from build123d import *

# Parameters (mm, degrees)
F0_R       = 17.0692141661
F1_DEPTH   = 74.676
F3_DEPTH   = 7.62
F1_FACE1_R = 17.0692141661
F5_DEPTH   = 8.128
F7_DEPTH   = 14.732
F9_DEPTH   = 14.478
F10_R      = 6.1442753349
F11_DEPTH  = 157.481
F12_R      = 6.3140721671
F13_DEPTH  = 157.481


with BuildPart() as f1:
    # F0 (on Right) → F1 (new body, symmetric)
    with BuildSketch(Plane.YZ):
        with Locations((0, -44.9254028499)):
            Circle(F0_R)
    extrude(amount=F1_DEPTH, both=True)

    # F2 (on face) → F3 (join)
    with BuildSketch(Plane.YZ.offset(74.676)):
        with BuildLine():
            ThreePointArc((17.0692141661, -44.9254028499), (17.054567773, -45.6323613518), (17.0106537288, -46.3381066294))
            Line((17.0106537288, -46.3381066294), (17.6849197596, -46.3381066294))
            Line((17.6849197596, -46.3381066294), (17.6849197596, 24.6733147651))
            Line((17.6849197596, 24.6733147651), (-17.0106537288, 24.6733147651))
            Line((-17.0106537288, 24.6733147651), (-17.0106537288, -43.5126990704))
            ThreePointArc((-17.0106537288, -43.5126990704), (0.7069585019, -27.8708350769), (17.0692141661, -44.9254028499))
        make_face()
    extrude(amount=-F3_DEPTH)

    # F4 (on face) + F1_face1 (on face) → F5 (join)
    with BuildSketch(Plane.YZ.offset(74.676)):
        with BuildLine():
            Line((-17.0106537288, 24.6733147651), (17.6849197596, 24.6733147651))
            ThreePointArc((17.6849197596, 24.6733147651), (0.3371330154, 42.0211015093), (-17.0106537288, 24.6733147651))
        make_face()
    with BuildSketch(Plane(origin=(-74.676, 0, -44.9254028499), x_dir=(0, 1, 0), z_dir=(-1, 0, 0))):
        Circle(F1_FACE1_R)
    extrude(amount=-F5_DEPTH, dir=(1, 0, 0))

    # F6 (on face) → F7 (join)
    with BuildSketch(Plane(origin=(-82.804, 0, 0), x_dir=(0, -1, 0), z_dir=(-1, 0, 0))):
        with BuildLine():
            ThreePointArc((17.0692141661, -44.9254028499), (17.0670540007, -45.1969539267), (17.060574051, -45.4684362721))
            Line((17.060574051, -45.4684362721), (17.1144399792, -45.4684362721))
            Line((17.1144399792, -45.4684362721), (17.1144399792, 24.6733147651))
            Line((17.1144399792, 24.6733147651), (-17.060574051, 24.6733147651))
            Line((-17.060574051, 24.6733147651), (-17.060574051, -44.3823694277))
            ThreePointArc((-17.060574051, -44.3823694277), (0.2715510768, -27.8583488493), (17.0692141661, -44.9254028499))
        make_face()
    extrude(amount=-F7_DEPTH)

    # F8 (on face) → F9 (join)
    with BuildSketch(Plane(origin=(-82.804, 0, 0), x_dir=(0, -1, 0), z_dir=(-1, 0, 0))):
        with BuildLine():
            Line((-17.060574051, 24.6733147651), (17.1144399792, 24.6733147651))
            ThreePointArc((17.1144399792, 24.6733147651), (0.0269329641, 41.7608217802), (-17.060574051, 24.6733147651))
        make_face()
    extrude(amount=-F9_DEPTH)

    # F10 (on face) → F11 (cut, through all)
    with BuildSketch(Plane.YZ.offset(74.676)):
        with Locations((0, -49.4892522693)):
            Circle(F10_R)
    extrude(amount=-F11_DEPTH, mode=Mode.SUBTRACT)

    # F12 (on face) → F13 (cut, through all)
    with BuildSketch(Plane.YZ.offset(74.676)):
        with Locations((0, 31.5190926194)):
            Circle(F12_R)
    extrude(amount=-F13_DEPTH, mode=Mode.SUBTRACT)


solid = f1.part
Build history of the part. All positions in model axes, mm. A direction names the side the tool comes from. Round coordinates to 2 decimals unless told otherwise and drop trailing zeros. Write each loop counter-clockwise with the first axis right and the second up, starting at its lowest first coordinate (ties: lowest second). Pieces come first, ordered by that corner, then holes. Notation, with made-up numbers: (17, -33) - (46, -33) arc R24 cw to (46, -8) - close; hole circle Ø1 at (70, 74). An arc over 180 degrees is marked (long way). Use CSV: the item, a comma, the result in double quotes.
(1) Band-saw the part on A-A (z = -16). Write the cut outline in (x, y).
Response:
outline,"(-82.8, -17.11) - (-68.07, -17.11) - (-68.07, 17.06) - (-82.8, 17.06) - close; (67.06, -17.01) - (74.68, -17.01) - (74.68, 17.68) - (67.06, 17.68) - close"
(2) Band-saw the part on B-B (y = 0). Write the cut outline in (x, z), plus the area to 3 significant figures.
Response:
outline,"(-82.8, -61.99) - (74.68, -61.99) - (74.68, -55.63) - (-82.8, -55.63) - close; (-82.8, -43.34) - (74.68, -43.34) - (74.68, 25.21) - (66.55, 25.21) - (66.55, 24.67) - (67.06, 24.67) - (67.06, -27.86) - (-68.07, -27.86) - (-68.07, 24.67) - (-68.33, 24.67) - (-68.33, 25.21) - (-82.8, 25.21) - close; (-82.8, 37.83) - (-68.33, 37.83) - (-68.33, 41.76) - (-82.8, 41.76) - close; (66.55, 37.83) - (74.68, 37.83) - (74.68, 42.02) - (66.55, 42.02) - close"
area,"4,720 mm²"
(3) Band-saw the part on C-C (x = -28). Write the cut outline in (y, z), plus the area to 3 significant figures.
Response:
outline,"circle Ø34.14 at (0, -44.93); hole circle Ø12.29 at (0, -49.49)"
area,"797 mm²"
(4) Mould opens along Z. For faces 1 (the cylindrical face through (70.669, 0.719, 42.017)), 2 (the cylindrical face through (70.669, -1.369, 25.355)), 3 (the flat face through (66.548, 4, 37)) say: pulls with the +Z half, pulls with the -Z half, needs draft (parallel to the pull), parting line crosses it, or undercut.
Response:
face 1,"pulls with the +Z half"
face 2,"undercut"
face 3,"needs draft"
(5) Band-saw the part on D-D (y = -12). Write the cut outline in (x, z).
Response:
outline,"(-82.8, -57.06) - (74.68, -57.06) - (74.68, 36.87) - (66.55, 36.87) - (66.55, 24.67) - (67.06, 24.67) - (67.06, -32.79) - (-68.07, -32.79) - (-68.07, 24.67) - (-68.33, 24.67) - (-68.33, 36.86) - (-82.8, 36.86) - close"
(6) 3-axis set-ups, long thin cutter, end or side, ignore diameter. For faces 4 (the flat face through (-68.326, -4, 37)), 5 (the cylindrical face through (-2.96, -3.7, -61.59)), 6 (the flat face through (-76, 17.061, -9)), 7 (the cylindrical face through (-75.666, -0.403, 41.757)): which of +Z, -Z, +X, -X, +Y, -Y reach the whole face in a straight line?
Response:
face 4,"+Z, +Y, -Y"
face 5,"none"
face 6,"+Z, -Z, -X, +Y"
face 7,"+Z, -X"
(7) Wall check: line 1 (Z direction, x = 68.5, y = 0); line 2 (X direction, y = 16.5, z = 4); line 3 (Z direction, x = -27, y = 0). Give the ranges that are in metal, low to high.
Response:
line 1,"-61.99 to -55.63, -43.34 to 25.21, 37.83 to 42.02"
line 2,"-82.8 to -68.07, 67.06 to 74.68"
line 3,"-61.99 to -55.63, -43.34 to -27.86"
(8) Pin check, flat tips, straight feed: P1, Ø5, axis at x = 3.5, y = -11.5, coming from the +Z side; P2, Ø4, axis at x = 71, z = -3.5, coming from the -Y side; P3, Ø3, axis at x = -35.5, y = 4, coming from the +Z side; P4, Ø5, axis at y = 1, z = 32.5, coming from the -X side. Stop position of each tip, or through.
Response:
P1,"z = -30.42"
P2,"y = -17.01"
P3,"z = -28.04"
P4,"through"
